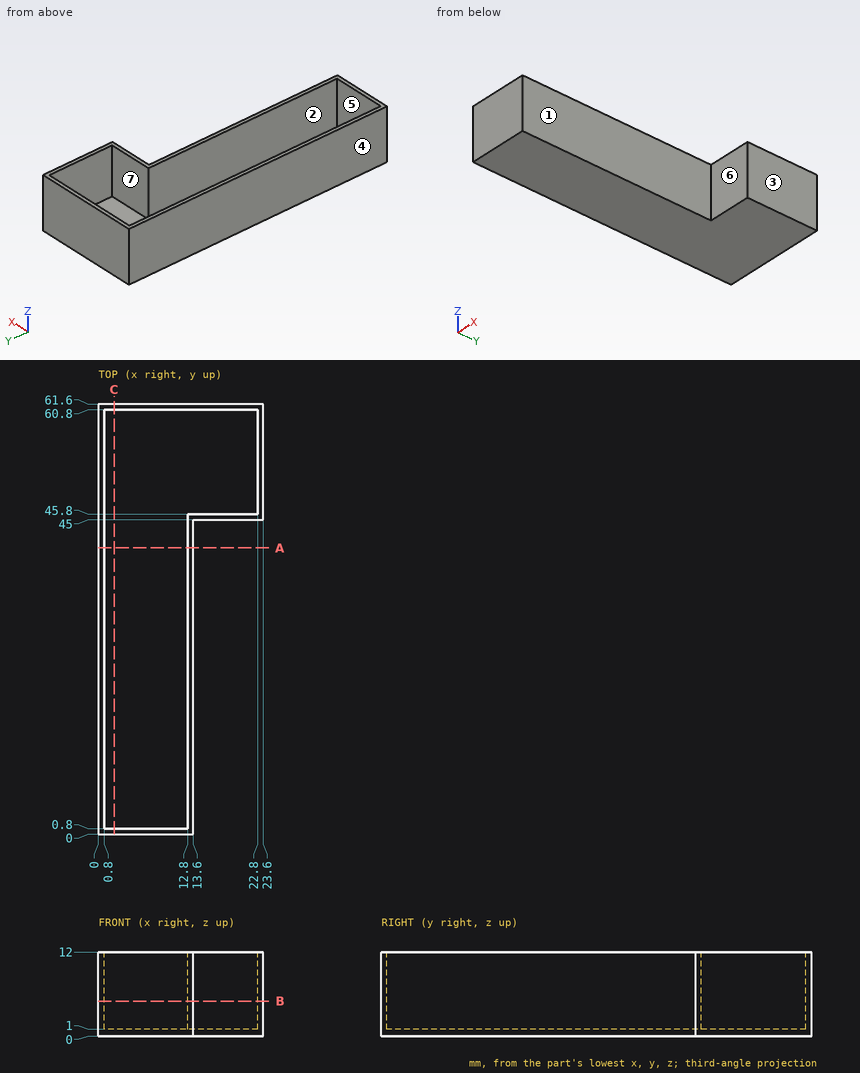
Can you work these out from the drawing? Everything is in mm from the part's minimum corner. A direction names the side the tool comes from. Give positions to 0.01 mm unless a question says otherwise; leave off trailing zeros. Order: outer loops, then holes, each group sorted by start corner. A loop starts at its lowest first (then second) coordinate and runs counter-clockwise, first axis right, second up.
Item 1: I'm going to push flat-ended pins straight in: pin 1 (6 mm diameter, centred on y = 26, z = 8.5, fed in from +X); pin 2 (1 mm diameter, centred on x = 18, z = 8, fed in from -Y); pin 3 (3 mm diameter, centred on x = 6.5, y = 33.5, fed in from +Z). Where does each tip first touch, or does it pass through?
Item 2: If we section it at B-B, the plane z = 5: Write out the boundary of the cut face in (x, y), plus the area to 3 significant figures.
Item 3: If we mould it in two halves opening along X, with no side actions, what happens to the marked faces 4, 5, 6 and 7? For each: pulls with the +X half, pulls with the -X half, needs draft (parallel to the pull), parting line crosses it, or undercut.
Item 4: If we section it at C-C, the plane x = 2.25: Write out the boundary of the cut face in (y, z).
Item 5: If we section it at A-A, the plane y = 41: Write out the boundary of the cut face in (x, z), plus the area to 3 significant figures.
Item 6: I need wall thicknesses on line 1 (Y direction, x = 3, z = 7.75); line 2 (X direction, y = 30, z = 2.75); line 3 (Y direction, x = 13, z = 2.5). Which ranges of each line are inside material? Lowest first, please.
Item 7: For the marked faces 1, 2 and 3, which set-ups out of +Z, -Z, +X, -X, +Y, -Y let a thin tool reach every point of the face, with its end or its side?
Values:
1. pin 1: stops at x = 13.6
1. pin 2: stops at y = 45
1. pin 3: stops at z = 1
2. outline: (0, 0) - (13.6, 0) - (13.6, 45) - (23.6, 45) - (23.6, 61.6) - (0, 61.6) - close; hole (0.8, 0.8) - (12.8, 0.8) - (12.8, 45.8) - (22.8, 45.8) - (22.8, 60.8) - (0.8, 60.8) - close
2. area: 134 mm2
3. face 4: pulls with the -X half
3. face 5: undercut
3. face 6: needs draft
3. face 7: undercut
4. outline: (0, 0) - (61.6, 0) - (61.6, 12) - (60.8, 12) - (60.8, 1) - (0.8, 1) - (0.8, 12) - (0, 12) - close
5. outline: (0, 0) - (13.6, 0) - (13.6, 12) - (12.8, 12) - (12.8, 1) - (0.8, 1) - (0.8, 12) - (0, 12) - close
5. area: 31.2 mm2
6. line 1: y = 0 to 0.8, 60.8 to 61.6
6. line 2: x = 0 to 0.8, 12.8 to 13.6
6. line 3: y = 0 to 45.8, 60.8 to 61.6
7. face 1: +Z, -Z, +X, -Y
7. face 2: +Z
7. face 3: +Z, -Z, +X, +Y, -Y
